Can you work these out from the model? Positions are in its coordinate system, mm. Face numbers are marked on the shaded views. A direction names the side the tool comes from. Coordinates: 2 decimals unless noted, no trailing zeros. Loops run counter-clockwise (first coordinate to the right, second up) from the corner with the lowest first, then second, coordinate; pieces in that order, holes last. Notation, with made-up numbers: M 73,1.25 L 126,1.25 A19 ccw 126,34.25 Z; hole C 27,82.25 d9. An arc over 180 degrees is marked long. Return JSON: item names as keys, results as strings. Group by question number.
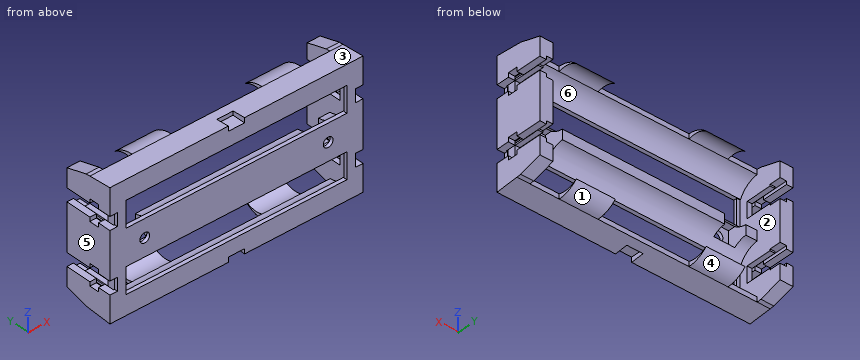
```python
from build123d import *

# Parameters (mm, degrees)
SKETCH1_W            = 78
SKETCH1_H            = 39
BOSS_EXTRUDE1_DEPTH  = 7
CUT_EXTRUDE1_DEPTH   = 81.704708661
SKETCH3_W            = 70
SKETCH3_H            = 8
CUT_EXTRUDE2_DEPTH   = 6
CUT_EXTRUDE3_DEPTH   = 70
MIRROR9_COPY_1_DEPTH = 70
MIRROR9_COPY_2_DEPTH = 70
SKETCH5_W            = 68
SKETCH5_H            = 8
CUT_EXTRUDE4_DEPTH   = 45.014202253
BOSS_EXTRUDE2_DEPTH  = 12
MIRROR3_COPY_1_DEPTH = 12
BOSS_EXTRUDE3_DEPTH  = 4
SKETCH9_W            = 6.5
SKETCH9_H            = 3
CUT_EXTRUDE5_DEPTH   = 2
CUT_EXTRUDE6_DEPTH   = 2
SKETCH12_W           = 0.5
SKETCH12_H           = 6
CUT_EXTRUDE11_DEPTH  = 10.5
SKETCH13_W           = 4.001855858
SKETCH13_H           = 15
CUT_EXTRUDE9_DEPTH   = 2.3
SKETCH14_W           = 5
SKETCH14_H           = 1.5
CUT_EXTRUDE10_DEPTH  = 4
SKETCH15_W           = 6.5
SKETCH15_H           = 6
CUT_EXTRUDE12_DEPTH  = 6
CUT_EXTRUDE13_REACH  = 47.796
SKETCH16_R           = 1.5


with BuildPart() as part:
    # Sketch1 → Boss-Extrude1 (new body)
    with BuildSketch(Plane(origin=(0, 0, 0), x_dir=(1, 0, 0), z_dir=(0, 1, 0))):
        Rectangle(SKETCH1_W, SKETCH1_H)
    extrude(amount=BOSS_EXTRUDE1_DEPTH)

    # Sketch2 → Cut-Extrude1 (cut, through all)
    with BuildSketch(Plane(origin=(39, 0, 0), x_dir=(0, 0, -1), z_dir=(1, 0, 0))):
        Polygon((19, 7), (19.5, 0), (19.5, 7), align=None)
        Polygon((-19, 7), (-19.5, 0), (-19.5, 7), align=None)
    extrude(amount=-CUT_EXTRUDE1_DEPTH, mode=Mode.SUBTRACT)

    # Sketch3 → Cut-Extrude2 (cut)
    with BuildSketch(Plane(origin=(0, 7, 0), x_dir=(1, 0, 0), z_dir=(0, 1, 0))):
        with Locations((0, -9.5)):
            Rectangle(SKETCH3_W, SKETCH3_H)
        with Locations((0, 9.5)):
            Rectangle(SKETCH3_W, SKETCH3_H)
    extrude(amount=-CUT_EXTRUDE2_DEPTH, mode=Mode.SUBTRACT)

    # Sketch4 → Cut-Extrude3 (cut)
    with BuildSketch(Plane(origin=(35, 0, 0), x_dir=(0, 0, -1), z_dir=(1, 0, 0))):
        with BuildLine():
            Line((13, 1), (13, 7))
            Line((13, 7), (17.5, 7))
            ThreePointArc((17.5, 7), (16.132310367, 3.338267225), (13, 1))
        make_face()
    cut_extrude3 = extrude(amount=-CUT_EXTRUDE3_DEPTH, mode=Mode.SUBTRACT)

    # Mirror1: Cut-Extrude3 across plane
    add(cut_extrude3.mirror(Plane.XY), mode=Mode.SUBTRACT)

    # Mirror8: Cut-Extrude3 across plane
    add(cut_extrude3.mirror(Plane.XY.offset(-9.5)), mode=Mode.SUBTRACT)

    # Mirror9 copy 1 sketch → Mirror9 copy 1 (cut)
    with BuildSketch(Plane(origin=(35, 0, 19), x_dir=(0, 0, -1), z_dir=(1, 0, 0))):
        with BuildLine():
            Line((13, 1), (13, 7))
            Line((13, 7), (17.5, 7))
            ThreePointArc((17.5, 7), (16.132310367, 3.338267225), (13, 1))
        make_face()
    extrude(amount=-MIRROR9_COPY_1_DEPTH, mode=Mode.SUBTRACT)

    # Mirror9 copy 2 sketch → Mirror9 copy 2 (cut)
    with BuildSketch(Plane(origin=(35, 0, 19), x_dir=(0, 0, 1), z_dir=(1, 0, 0))):
        with BuildLine():
            Line((13, -1), (13, -7))
            Line((13, -7), (17.5, -7))
            ThreePointArc((17.5, -7), (16.132310367, -3.338267225), (13, -1))
        make_face()
    extrude(amount=-MIRROR9_COPY_2_DEPTH, mode=Mode.SUBTRACT)

    # Sketch5 → Cut-Extrude4 (cut, through all)
    with BuildSketch(Plane(origin=(0, 1, 0), x_dir=(1, 0, 0), z_dir=(0, 1, 0))):
        with Locations((0, 9.5)):
            Rectangle(SKETCH5_W, SKETCH5_H)
        with Locations((0, -9.5)):
            Rectangle(SKETCH5_W, SKETCH5_H)
    extrude(amount=-CUT_EXTRUDE4_DEPTH, mode=Mode.SUBTRACT)

    # Sketch6 → Boss-Extrude2 (add)
    with BuildSketch(Plane(origin=(26, 0, 0), x_dir=(0, 0, -1), z_dir=(1, 0, 0))):
        with BuildLine():
            Line((-19, 7), (-17.5, 7))
            ThreePointArc((-17.5, 7), (-17.740958247, 10.123493041), (-16.5, 13))
            ThreePointArc((-16.5, 13), (-18.343954985, 10.247481244), (-19, 7))
        make_face()
    boss_extrude2 = extrude(amount=-BOSS_EXTRUDE2_DEPTH)

    # Mirror2: Boss-Extrude2 across plane
    add(boss_extrude2.mirror(Plane(origin=(0, 0, 0), x_dir=(0, 0, 1), z_dir=(1, 0, 0))))

    # Mirror3: Boss-Extrude2 across plane
    add(boss_extrude2.mirror(Plane.XY))

    # Mirror3 copy 1 sketch → Mirror3 copy 1 (add)
    with BuildSketch(Plane.ZY.offset(26)):
        with BuildLine():
            Line((-19, 7), (-17.5, 7))
            ThreePointArc((-17.5, 7), (-17.740958247, 10.123493041), (-16.5, 13))
            ThreePointArc((-16.5, 13), (-18.343954985, 10.247481244), (-19, 7))
        make_face()
    extrude(amount=-MIRROR3_COPY_1_DEPTH)

    # Sketch8 → Boss-Extrude3 (add)
    with BuildSketch(Plane(origin=(39, 0, 0), x_dir=(0, 0, -1), z_dir=(1, 0, 0))):
        Polygon((-17, 15), (17, 15), (18.894572253, 8.304261216), (19, 7), (-19, 7), (-18.894572253, 8.304261216), align=None)
    boss_extrude3 = extrude(amount=-BOSS_EXTRUDE3_DEPTH)

    # Mirror4: Boss-Extrude3 across plane
    add(boss_extrude3.mirror(Plane(origin=(0, 0, 0), x_dir=(0, 0, 1), z_dir=(1, 0, 0))))

    # Sketch9 → Cut-Extrude5 (cut)
    with BuildSketch(Plane(origin=(39, 0, 0), x_dir=(0, 0, -1), z_dir=(1, 0, 0))):
        with Locations((9.25, 5.5)):
            Rectangle(SKETCH9_W, SKETCH9_H)
        with Locations((-9.25, 5.5)):
            Rectangle(SKETCH9_W, SKETCH9_H)
    cut_extrude5 = extrude(amount=-CUT_EXTRUDE5_DEPTH, mode=Mode.SUBTRACT)

    # Mirror5: Cut-Extrude5 across plane
    add(cut_extrude5.mirror(Plane(origin=(0, 0, 0), x_dir=(0, 0, 1), z_dir=(1, 0, 0))), mode=Mode.SUBTRACT)

    # Sketch11 → Cut-Extrude6 (cut)
    with BuildSketch(Plane.ZY.offset(-35)):
        Polygon((6.75, 3.5), (11.75, 3.5), (11.75, 11.5), (12.25, 11.5), (12.25, 15), (6.25, 15), (6.25, 11.5), (6.75, 11.5), align=None)
        Polygon((-6.75, 11.5), (-6.25, 11.5), (-6.25, 15), (-12.25, 15), (-12.25, 11.5), (-11.75, 11.5), (-11.75, 3.5), (-6.75, 3.5), align=None)
    cut_extrude6 = extrude(amount=-CUT_EXTRUDE6_DEPTH, mode=Mode.SUBTRACT)

    # Sketch12 → Cut-Extrude11 (cut)
    with BuildSketch(Plane(origin=(0, 11.5, 0), x_dir=(1, 0, 0), z_dir=(0, 1, 0))):
        with Locations((36.75, 9.25)):
            Rectangle(SKETCH12_W, SKETCH12_H)
        with Locations((36.75, -9.25)):
            Rectangle(SKETCH12_W, SKETCH12_H)
    cut_extrude11 = extrude(amount=-CUT_EXTRUDE11_DEPTH, mode=Mode.SUBTRACT)

    # Sketch13 → Cut-Extrude9 (cut)
    with BuildSketch(Plane(origin=(39, 0, 0), x_dir=(0, 0, -1), z_dir=(1, 0, 0))):
        with Locations((9.25, 7.5)):
            Rectangle(SKETCH13_W, SKETCH13_H)
        with Locations((-9.25, 7.5)):
            Rectangle(SKETCH13_W, SKETCH13_H)
    cut_extrude9 = extrude(amount=-CUT_EXTRUDE9_DEPTH, mode=Mode.SUBTRACT)

    # Mirror10: Cut-Extrude6, Cut-Extrude11, Cut-Extrude9 across plane
    add(cut_extrude6.mirror(Plane(origin=(0, 0, 0), x_dir=(0, 0, 1), z_dir=(1, 0, 0))), mode=Mode.SUBTRACT)
    add(cut_extrude11.mirror(Plane(origin=(0, 0, 0), x_dir=(0, 0, 1), z_dir=(1, 0, 0))), mode=Mode.SUBTRACT)
    add(cut_extrude9.mirror(Plane(origin=(0, 0, 0), x_dir=(0, 0, 1), z_dir=(1, 0, 0))), mode=Mode.SUBTRACT)

    # Sketch14 → Cut-Extrude10 (cut)
    with BuildSketch(Plane.XZ):
        with Locations((0, 18.75)):
            Rectangle(SKETCH14_W, SKETCH14_H)
    cut_extrude10 = extrude(amount=-CUT_EXTRUDE10_DEPTH, mode=Mode.SUBTRACT)

    # Mirror7: Cut-Extrude10 across plane
    add(cut_extrude10.mirror(Plane.XY), mode=Mode.SUBTRACT)

    # Sketch15 → Cut-Extrude12 (cut)
    with BuildSketch(Plane(origin=(0, 7, 0), x_dir=(1, 0, 0), z_dir=(0, 1, 0))):
        with Locations((-28.25, 0)):
            Rectangle(SKETCH15_W, SKETCH15_H)
        with Locations((28.25, 0)):
            Rectangle(SKETCH15_W, SKETCH15_H)
    extrude(amount=-CUT_EXTRUDE12_DEPTH, mode=Mode.SUBTRACT)

    # Sketch16 → Cut-Extrude13 (cut, up to next)
    with BuildSketch(Plane(origin=(0, 1, 0), x_dir=(1, 0, 0), z_dir=(0, 1, 0)), mode=Mode.PRIVATE) as cut_extrude13_sk1:
        with Locations(Location((-28.25, 0, 0), (0, 0, 270))):
            Circle(SKETCH16_R)
    cut_extrude13_tool1 = extrude(cut_extrude13_sk1.sketch, amount=-CUT_EXTRUDE13_REACH, mode=Mode.PRIVATE) & part.part
    # Sketch16 → Cut-Extrude13 (cut, up to next)
    with BuildSketch(Plane(origin=(0, 1, 0), x_dir=(1, 0, 0), z_dir=(0, 1, 0)), mode=Mode.PRIVATE) as cut_extrude13_sk2:
        with Locations(Location((28.25, 0, 0), (0, 0, 270))):
            Circle(SKETCH16_R)
    cut_extrude13_tool2 = extrude(cut_extrude13_sk2.sketch, amount=-CUT_EXTRUDE13_REACH, mode=Mode.PRIVATE) & part.part
    add(cut_extrude13_tool1.solids().sort_by_distance((-28.25, 1, 0))[0], mode=Mode.SUBTRACT)
    add(cut_extrude13_tool2.solids().sort_by_distance((28.25, 1, 0))[0], mode=Mode.SUBTRACT)


solid = part.part
```
1) If I drill on line 1 (X direction, y = 0.3, z = 0); line 2 (X direction, y = 2, z = 5); line 3 (Z direction, x = 18, y = 1), over which ranges is the centre line in solid material (lowest first)? Write a range as from..to.
2) If we mould it in two halves opening along Y, with no side actions, what happens to the marked faces 4, 5 and 6? For each: +Y half, -Y half, draft (parallel to the pull), parting line (faces both ways), or undercut.
3) Suppose I cut it at D-D, the plane y = 5.5. Give the number of separate pieces and of enclosed holes in the cut face, then the cut area to 3 significant figures.
4) Suppose I cut it at B-B, the plane x = -16. List the corners of the cut face in (y, z) for me.
5) Suppose I cut it at C-C, the plane x = -28.25. List the corners of the cut face in (y, z) for me, then the cut area to 3 significant figures.
6) For the marked faces 1, 2 and 3, which set-ups out of +Z, -Z, +X, -X, +Y, -Y let a thin tool reach every point of the face, with its end or its side?
7) For pin 1 (0.7 mm diameter, centred on x = 26.5, y = 2, fed in from -Z); pin 2 (2 mm diameter, centred on x = 38.5, y = 12, fed in from -Z); pin 3 (1 mm diameter, centred on x = -16.5, y = 2, fed in from +Z); pin 4 (1 mm diameter, centred on x = -8.5, y = 9, fed in from +Z), each with a flat end and sliding along its axis, tell me the tip position at first contact or that it passes through.
8) Suppose I cut it at A-A, the plane z = 0. List the corners of the cut face in (x, y) for me, then the cut area to 3 significant figures.
Returned:
{
 "1": {"line 1": "x = -39..-29.75, -26.75..26.75, 29.75..39", "line 2": "x = -39..-35, 35..39", "line 3": "z = -19.43..-13.5, -5.5..5.5, 13.5..19.43"},
 "2": {"face 4": "+Y half", "face 5": "draft", "face 6": "undercut"},
 "3": {"separate pieces": "5", "enclosed holes": "0", "area": "678 mm²"},
 "4": {"outline": "M 0,-19.5 L 7,-19 A8.53 ccw 13,-16.5 A6.53 cw 7,-17.5 A6.93 cw 1.21,-13.5 L 0,-13.5 Z; M 0,-5.5 L 1.21,-5.5 A6.93 cw 7,-1.5 L 7,1.5 A6.93 cw 1.21,5.5 L 0,5.5 Z; M 0,13.5 L 1.21,13.5 A6.93 cw 7,17.5 A6.53 cw 13,16.5 A8.53 ccw 7,19 L 0,19.5 Z"},
 "5": {"outline": "M 0,-19.5 L 7,-19 L 7,-17.5 A6.93 cw 1.21,-13.5 L 0,-13.5 Z; M 0,-5.5 L 1.21,-5.5 A6.93 cw 3.17,-3 L 1,-3 L 1,-1.5 L 0,-1.5 Z; M 0,1.5 L 1,1.5 L 1,3 L 3.17,3 A6.93 cw 1.21,5.5 L 0,5.5 Z; M 0,13.5 L 1.21,13.5 A6.93 cw 7,17.5 L 7,19 L 0,19.5 Z", "area": "61.3 mm²"},
 "6": {"face 1": "-Z, +Y", "face 2": "+Y", "face 3": "+Z, +X, -X, +Y"},
 "7": {"pin 1": "stops at z = -19.38", "pin 2": "stops at z = -18.13", "pin 3": "stops at z = 19.39", "pin 4": "passes through"},
 "8": {"outline": "M -39,0 L -29.75,0 L -29.75,1 L -31.5,1 L -31.5,7 L -35,7 L -35,15 L -39,15 Z; M -26.75,0 L 26.75,0 L 26.75,1 L 25,1 L 25,7 L -25,7 L -25,1 L -26.75,1 Z; M 29.75,0 L 39,0 L 39,15 L 35,15 L 35,7 L 31.5,7 L 31.5,1 L 29.75,1 Z", "area": "526 mm²"}
}
